Can you work these out from the model? Positions are in its coordinate system, mm. Coordinates: 2 decimals unless noted, no trailing zeros. Loops run counter-clockwise (first coordinate to the right, second up) from the corner with the lowest first, then second, coordinate; pieces in that order, holes last.
```python
from build123d import *

# Parameters (mm, degrees)
BOSS_EXTRUDE1_DEPTH = 4
CHAMFER1_SIZE       = 6
CHAMFER2_SIZE       = 2.6
CHAMFER2_SIZE2      = 4.5033321
SKETCH2_R           = 0.464535938
CUT_EXTRUDE1_DEPTH  = 0.5


with BuildPart() as part:
    # Sketch1 → Boss-Extrude1 (new body)
    with BuildSketch(Plane.XY):
        Polygon((0, 0), (20, 0), (20, 5), (0, 5), (0, 9), (-10, 9), (-10, 5), (-228.5, 5), (-228.5, 9), (-228.3, 9), (-228.5, 10.5), (-238.142857143, 10.5), (-241, 7.5), (-241, 6.475), (-236, 6.475), (-236, 8.5), (-235.5, 8.5), (-235.5, 7.75), (-233, 7.75), (-233, 6.475), (-232, 6.475), (-232, 3.525), (-233, 3.525), (-233, 2.25), (-235.5, 2.25), (-235.5, 1.5), (-236, 1.5), (-236, 3.525), (-241, 3.525), (-241, 2.5), (-240.8, 1.134476763), (-240.8, -0.5), (-245.2, -0.5), (-245.2, 2), (-249.093151184, 2), (-249.093151184, 5), (-285, 5), (-285, 9), (-295, 9), (-295, 5), (-289, -1), (-289, -10), (0, -10), align=None)
    extrude(amount=BOSS_EXTRUDE1_DEPTH)

    # Chamfer1
    chamfer1_edges = [part.edges().sort_by_distance(p)[0] for p in [
        (0, -10, 2),
    ]]
    chamfer(chamfer1_edges, length=CHAMFER1_SIZE)

    # Chamfer2
    chamfer2_edges = [part.edges().sort_by_distance(p)[0] for p in [
        (-249.093151184, 5, 2),
    ]]
    chamfer2_side = [part.faces().sort_by_distance(p)[0] for p in [
        (-249.093151184, 3.5, 2),
    ]]
    chamfer(chamfer2_edges, length=CHAMFER2_SIZE, length2=CHAMFER2_SIZE2, reference=chamfer2_side[0])

    # Sketch2 → Cut-Extrude1 (cut)
    with BuildSketch(Plane.ZY.offset(232)):
        with Locations((2, 5)):
            Circle(SKETCH2_R)
    extrude(amount=-CUT_EXTRUDE1_DEPTH, mode=Mode.SUBTRACT)


solid = part.part
```
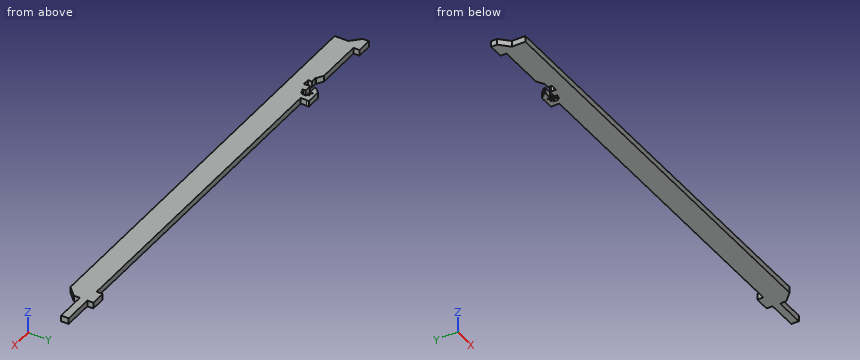
(1) If I drill on probe 1 along Y at (x, z) = (-231.7, 2); probe 2 along X at (y, z) = (8.75, 2.9); probe 3 along X at (y, z) = (-1.5, 1.65), over which ranges is the centre line in solid material (lowest first)?
Check values:
probe 1: y = -10 to 4.54, 5.46 to 10.5
probe 2: x = -295 to -285, -239.81 to -228.5, -10 to 0
probe 3: x = -289 to 0
(2) I'm going to push flat-ended pins straight in: pin 1 (12 mm diameter, centred on x = -255.5, y = -8, fed in from -Z); pin 2 (0.8 mm diameter, centred on y = 2, z = 1.5, fed in from -X); pin 3 (2 mm diameter, centred on x = -289, z = 1, fed in from +Y); pin 4 (1.4 mm diameter, centred on y = 2.5, z = 2, fed in from -X). Where does each tip first touch, or does it pass through?
Check values:
pin 1: stops at z = 0
pin 2: stops at x = -292.4
pin 3: stops at y = 9
pin 4: stops at x = -293.2
(3) I want a section at A-A on x = -116. Write out the boundary of the cut face in (y, z).
Check values:
outline: (-10, 0) - (5, 0) - (5, 4) - (-10, 4) - close
(4) I want a section at B-B on y = -7. Write out the boundary of the cut face in (x, z), then the cut area to 3 significant figures.
Check values:
outline: (-289, 0) - (-3, 0) - (-3, 4) - (-289, 4) - close
area: 1,140 mm2
